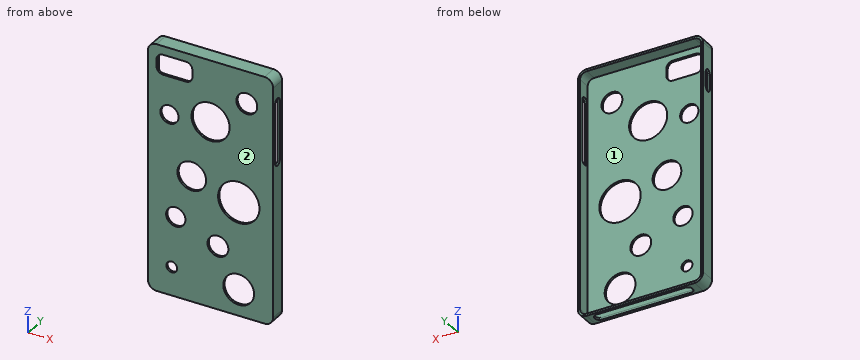
```python
from build123d import *

# Parameters (mm, degrees)
F0_W         = 73.66
F0_H         = 145.796
F1_DEPTH     = 8.89
F2_R         = 5.08
F3_W         = 21.0629868459
F3_H         = 11.8066714083
F4_DEPTH     = 12.7
F5_R         = 3.81
F7_T         = -1.27
F9_DEPTH     = 7.62
F10_W        = 4.164762795
F10_H        = 13.3272446692
F11_DEPTH    = 25.4
F12_T1_DEPTH = 1.27
F13_W        = 57.5663968921
F13_H        = 5.6068669073
F14_DEPTH    = 25.4
F15_R        = 2.54
F16_W        = 4.7923256643
F16_H        = 39.9060079362
F17_DEPTH    = 25.4
F18_T1_DEPTH = 1.27
F20_DEPTH    = 25.4
F21_R        = 12.1645390549
F21_R_2      = 8.4445659424
F21_R_3      = 5.6782177744
F21_R_4      = 6.1332477191
F21_R_5      = 9.0595333528
F21_R_6      = 3.1849618728
F21_R_7      = 5.3665907278
F21_R_8      = 6.1379255293
F22_DEPTH    = 25.4


# Not quite as in the source:
# - a fillet or chamfer that OpenCascade refuses, or shapes differently, is made with other operations: its cross-section is extruded or revolved along the edge and cut away or added


with BuildPart() as f1:
    # F0 (on Front) → F1 (new body)
    with BuildSketch(Plane.XZ):
        with Locations((-5.763799886, -17.0958732503)):
            Rectangle(F0_W, F0_H)
    extrude(amount=F1_DEPTH)

    # F2
    f2_edges = [f1.edges().sort_by_distance(p)[0] for p in [
        (31.0662, -4.445, 55.802127),
        (-42.5938, -4.445, 55.802127),
        (31.0662, -4.445, -89.993873),
        (-42.5938, -4.445, -89.993873),
    ]]
    fillet(f2_edges, radius=F2_R)

    # F3 (on face) → F4 (cut, symmetric)
    with BuildSketch(Plane.XZ.offset(8.89)):
        with Locations((-26.9823064631, 44.8187910455)):
            Rectangle(F3_W, F3_H)
    extrude(amount=F4_DEPTH, both=True, mode=Mode.SUBTRACT)

    # F5
    f5_edges = [f1.edges().sort_by_distance(p)[0] for p in [
        (-16.450813, -4.445, 50.722127),
        (-37.5138, -4.445, 50.722127),
        (-37.5138, -4.445, 38.915455),
        (-16.450813, -4.445, 38.915455),
    ]]
    fillet(f5_edges, radius=F5_R)

    # F7
    f7_openings = [f1.faces().sort_by_distance(p)[0] for p in [
        (-5.285571, 0, -18.491325),
    ]]
    offset(amount=F7_T, openings=f7_openings)

    # F8 (on face) → F9 (cut)
    with BuildSketch(Plane(origin=(0, 0, 0), x_dir=(-1, 0, 0), z_dir=(0, 1, 0))):
        Polygon((23.2353508472, 53.487226367), (11.2448604777, 51.826223731), (11.2448604777, 31.8353585899), (37.2746288776, 33.5012637079), (40.1331484318, 42.7181646228), (38.7322939932, 52.0863756537), align=None)
    extrude(amount=-F9_DEPTH, mode=Mode.SUBTRACT)

    # F10 (on face) → F11 (cut)
    with BuildSketch(Plane(origin=(-42.593799886, 0, 0), x_dir=(0, -1, 0), z_dir=(-1, 0, 0))):
        with Locations((4.5812404715, 30.585931614)):
            Rectangle(F10_W, F10_H)
    extrude(amount=-F11_DEPTH, mode=Mode.SUBTRACT)

    # F12: fillet of radius 2.54 on 4 edges, made by hand

    # F12_s2 → F12_t1 (join)
    with BuildSketch(Plane.YZ.offset(-42.593799886)):
        with BuildLine():
            ThreePointArc((-6.6636218689, 34.7095539486), (-5.9196730932, 36.5056051729), (-4.1236218689, 37.2495539486))
            Line((-4.1236218689, 37.2495539486), (-6.6636218689, 37.2495539486))
            Line((-6.6636218689, 37.2495539486), (-6.6636218689, 34.7095539486))
        make_face()
        with BuildLine():
            ThreePointArc((-6.6636218689, 26.4623092794), (-5.9196730932, 24.6662580552), (-4.1236218689, 23.9223092794))
            Line((-4.1236218689, 23.9223092794), (-6.6636218689, 23.9223092794))
            Line((-6.6636218689, 23.9223092794), (-6.6636218689, 26.4623092794))
        make_face()
        with BuildLine():
            ThreePointArc((-2.498859074, 34.7095539486), (-3.2428078498, 36.5056051729), (-5.038859074, 37.2495539486))
            Line((-5.038859074, 37.2495539486), (-2.498859074, 37.2495539486))
            Line((-2.498859074, 37.2495539486), (-2.498859074, 34.7095539486))
        make_face()
        with BuildLine():
            ThreePointArc((-5.038859074, 23.9223092794), (-3.2428078498, 24.6662580552), (-2.498859074, 26.4623092794))
            Line((-2.498859074, 26.4623092794), (-2.498859074, 23.9223092794))
            Line((-2.498859074, 23.9223092794), (-5.038859074, 23.9223092794))
        make_face()
    extrude(amount=F12_T1_DEPTH)

    # F13 (on face) → F14 (cut)
    with BuildSketch(Plane(origin=(0, 0, -89.9938732503), x_dir=(1, 0, 0), z_dir=(0, 0, -1))):
        with Locations((-5.0962045789, 4.3330059852)):
            Rectangle(F13_W, F13_H)
    extrude(amount=-F14_DEPTH, mode=Mode.SUBTRACT)

    # F15
    f15_edges = [f1.edges().sort_by_distance(p)[0] for p in [
        (-33.879403, -7.136439, -89.358873),
        (23.686994, -7.136439, -89.358873),
        (-33.879403, -1.529573, -89.358873),
        (23.686994, -1.529573, -89.358873),
    ]]
    fillet(f15_edges, radius=F15_R)

    # F16 (on face) → F17 (cut)
    with BuildSketch(Plane.YZ.offset(31.066200114)):
        with Locations((-4.6495434362, 22.6213793503)):
            Rectangle(F16_W, F16_H)
    extrude(amount=-F17_DEPTH, mode=Mode.SUBTRACT)

    # F18: fillet of radius 2.54 on 4 edges, made by hand

    # F18_s2 → F18_t1 (join)
    with BuildSketch(Plane.YZ.offset(29.796200114)):
        with BuildLine():
            ThreePointArc((-4.7933806041, 42.5743833184), (-2.9973293799, 41.8304345426), (-2.2533806041, 40.0343833184))
            Line((-2.2533806041, 40.0343833184), (-2.2533806041, 42.5743833184))
            Line((-2.2533806041, 42.5743833184), (-4.7933806041, 42.5743833184))
        make_face()
        with BuildLine():
            ThreePointArc((-2.2533806041, 5.2083753822), (-2.9973293799, 3.412324158), (-4.7933806041, 2.6683753822))
            Line((-4.7933806041, 2.6683753822), (-2.2533806041, 2.6683753822))
            Line((-2.2533806041, 2.6683753822), (-2.2533806041, 5.2083753822))
        make_face()
        with BuildLine():
            ThreePointArc((-4.5057062684, 42.5743833184), (-6.3017574926, 41.8304345426), (-7.0457062684, 40.0343833184))
            Line((-7.0457062684, 40.0343833184), (-7.0457062684, 42.5743833184))
            Line((-7.0457062684, 42.5743833184), (-4.5057062684, 42.5743833184))
        make_face()
        with BuildLine():
            ThreePointArc((-4.5057062684, 2.6683753822), (-6.3017574926, 3.412324158), (-7.0457062684, 5.2083753822))
            Line((-7.0457062684, 5.2083753822), (-7.0457062684, 2.6683753822))
            Line((-7.0457062684, 2.6683753822), (-4.5057062684, 2.6683753822))
        make_face()
    extrude(amount=F18_T1_DEPTH)

    # F19 (on face) → F20 (cut)
    with BuildSketch(Plane.XZ.offset(8.89)):
        with BuildLine():
            Line((-5.763799886, 8.3429517969), (-5.763799886, 30.7556648925))
            ThreePointArc((-5.763799886, 30.7556648925), (-16.9701564338, 19.5493083447), (-5.763799886, 8.3429517969))
        make_face()
        with BuildLine():
            ThreePointArc((5.4425566618, 19.5493083447), (2.1602908213, 27.473399052), (-5.763799886, 30.7556648925))
            Line((-5.763799886, 30.7556648925), (-5.763799886, 8.3429517969))
            ThreePointArc((-5.763799886, 8.3429517969), (2.1602908213, 11.6252176374), (5.4425566618, 19.5493083447))
        make_face()
    extrude(amount=-F20_DEPTH, mode=Mode.SUBTRACT)

    # F21 (on face) → F22 (cut)
    with BuildSketch(Plane.XZ.offset(8.89)):
        with Locations((10.8195273206, -23.030474782)):
            Circle(F21_R)
        with Locations((-16.8110914528, -15.915196389)):
            Circle(F21_R_2)
        with Locations((-26.2109395117, -42.8681261837)):
            Circle(F21_R_3)
        with Locations((-1.4226717176, -52.5855049491)):
            Circle(F21_R_4)
        with Locations((10.7564115897, -74.5054781437)):
            Circle(F21_R_5)
        with Locations((-28.563728556, -73.1163173914)):
            Circle(F21_R_6)
        with Locations((-29.9305599183, 16.5542345494)):
            Circle(F21_R_7)
        with Locations((15.5416298658, 36.8061438203)):
            Circle(F21_R_8)
    extrude(amount=-F22_DEPTH, mode=Mode.SUBTRACT)


solid = f1.part
```
Source: CAD feature listing. Evaluate the final solid. Frame: model axes, mm. Face numbers are marked on the shaded views. Give positions to 0.01 mm unless a question says otherwise; leave off trailing zeros. Loops run counter-clockwise (first coordinate to the right, second up) from the corner with the lowest first, then second, coordinate; pieces in that order, holes last. Notation, with made-up numbers: (-4, 33.25) -> (3, 33.25) arc R24 ccw to (3, 68.25) -> close; hole circle Ø6 at (83.25, -34). An arc over 180 degrees is marked (long way). Use a Markdown table: item, result. Add a question column.
(1) Section query B-B (z = -4.5). Output: boundary loops of the cut face in (x, y).
(2) Pull-direction query (X, two-part tool) for the marked faces 1 and 2; classes: +X half, -X half, draft (parallel to the pull), parting line (faces both ways), or undercut.
(3) Ray query, line 1 (Z direction, x = -34, y = -7); line 2 (X direction, y = -2.25, z = -65); line 3 (X direction, y = -5.5, z = 20). Return the intervals inside material, ascending.
(4) Section query A-A (z = -39). Output: boundary loops of the cut face in (x, y), then the cut area to 3 significant figures.
(5) Section query C-C (x = 11). Output: boundary loops of the cut face in (y, z).
(6) Section query D-D (z = -21.5). Output: boundary loops of the cut face in (x, y).
(7) First-contact query: pin 1 Ø10 at (x, z) = (-1.42, -52.59) entering from +Y; pin 2 Ø2 at (x, z) = (4, 12.5) entering from +Y. Flat tips, straight axial feed; report the tip coordinate or a pass-through.
Checked values:
| question | item | result |
|---|---|---|
| 1 | outline | (-42.59, -8.89) -> (31.07, -8.89) -> (31.07, 0) -> (29.8, 0) -> (29.8, -7.62) -> (-41.32, -7.62) -> (-41.32, 0) -> (-42.59, 0) -> close |
| 2 | face 1 | undercut |
| 2 | face 2 | draft |
| 3 | line 1 | -89.99 to -88.72, 54.53 to 55.8 |
| 3 | line 2 | -42.59 to -41.32, 29.8 to 31.07 |
| 3 | line 3 | -42.59 to -41.32 |
| 4 | outline | (-42.59, -8.89) -> (-30.37, -8.89) -> (-30.37, -7.62) -> (-41.32, -7.62) -> (-41.32, 0) -> (-42.59, 0) -> close; (-22.05, -8.89) -> (31.07, -8.89) -> (31.07, 0) -> (29.8, 0) -> (29.8, -7.62) -> (-22.05, -7.62) -> close |
| 4 | area | 102 mm^2 |
| 5 | outline | (-8.89, -89.99) -> (-7.14, -89.99) -> (-7.14, -88.72) -> (-7.62, -88.72) -> (-7.62, -83.56) -> (-8.89, -83.56) -> close; (-8.89, -65.45) -> (-7.62, -65.45) -> (-7.62, -35.19) -> (-8.89, -35.19) -> close; (-8.89, -10.87) -> (-7.62, -10.87) -> (-7.62, 32.68) -> (-8.89, 32.68) -> close; (-8.89, 40.94) -> (-7.62, 40.94) -> (-7.62, 54.53) -> (0, 54.53) -> (0, 55.8) -> (-8.89, 55.8) -> close; (-1.53, -89.99) -> (0, -89.99) -> (0, -88.72) -> (-1.53, -88.72) -> close |
| 6 | outline | (-42.59, -8.89) -> (-23.15, -8.89) -> (-23.15, -7.62) -> (-41.32, -7.62) -> (-41.32, 0) -> (-42.59, 0) -> close; (-10.48, -8.89) -> (-1.25, -8.89) -> (-1.25, -7.62) -> (-10.48, -7.62) -> close; (22.89, -8.89) -> (31.07, -8.89) -> (31.07, 0) -> (29.8, 0) -> (29.8, -7.62) -> (22.89, -7.62) -> close |
| 7 | pin 1 | through |
| 7 | pin 2 | y = -7.62 |
